Can you work these out from the model? Positions are in its coordinate system, mm. Face numbers are marked on the shaded views. Round coordinates to 2 decimals unless told otherwise and drop trailing zeros. Loops run counter-clockwise (first coordinate to the right, second up) from the corner with the lowest first, then second, coordinate; pieces in that order, holes last. Notation, with made-up numbers: (-18.5, -22) -> (14.5, -22) arc R13 ccw to (14.5, -8) -> close; hole circle Ø2 at (72, 18). An arc over 180 degrees is marked (long way). Use a Markdown table: item, result.
from build123d import *

# Parameters (mm, degrees)
F0_R     = 11.2
F0_R_2   = 13.2
F1_DEPTH = 7


with BuildPart() as f1:
    # F0 (on Top) → F1 (new body)
    with BuildSketch(Plane.XY):
        with BuildLine():
            ThreePointArc((10.232901, 19.541287), (12.436123, 23.454365), (13.2, 27.879616))
            ThreePointArc((13.2, 27.879616), (-4.186254, 40.398213), (-10.544739, 19.939308))
            ThreePointArc((-10.544739, 19.939308), (-0.252816, 14.682038), (10.232901, 19.541287))
        make_face()
        with Locations((0, 27.879616)):
            Circle(F0_R, mode=Mode.SUBTRACT)
        with BuildLine():
            ThreePointArc((-10.944456, -13.939808), (-14.094014, -5.382436), (-22.039701, -0.908691))
            ThreePointArc((-22.039701, -0.908691), (-35.700302, -20.319652), (-11.995578, -19.101666))
            ThreePointArc((-11.995578, -19.101666), (-11.209906, -16.573704), (-10.944456, -13.939808))
        make_face()
        with Locations((-24.144456, -13.939808)):
            Circle(F0_R, mode=Mode.SUBTRACT)
        with BuildLine():
            ThreePointArc((37.344456, -13.939808), (32.892752, -4.055107), (22.540317, -0.837643))
            ThreePointArc((22.540317, -0.837643), (12.841425, -7.122074), (11.8068, -18.632596))
            ThreePointArc((11.8068, -18.632596), (26.530137, -26.922432), (37.344456, -13.939808))
        make_face()
        with Locations((24.144456, -13.939808)):
            Circle(F0_R, mode=Mode.SUBTRACT)
        with BuildLine():
            ThreePointArc((10.232901, 19.541287), (-0.252816, 14.682038), (-10.544739, 19.939308))
            ThreePointArc((-10.544739, 19.939308), (-11.60274, 6.92967), (-22.039701, -0.908691))
            ThreePointArc((-22.039701, -0.908691), (-14.094014, -5.382436), (-10.944456, -13.939808))
            ThreePointArc((-10.944456, -13.939808), (-11.209906, -16.573704), (-11.995578, -19.101666))
            ThreePointArc((-11.995578, -19.101666), (-0.1999, -13.513102), (11.8068, -18.632596))
            ThreePointArc((11.8068, -18.632596), (12.841425, -7.122074), (22.540317, -0.837643))
            ThreePointArc((22.540317, -0.837643), (11.80264, 6.583433), (10.232901, 19.541287))
        make_face()
        Circle(F0_R_2, mode=Mode.SUBTRACT)
        Circle(F0_R_2)
        Circle(F0_R, mode=Mode.SUBTRACT)
    extrude(amount=F1_DEPTH)


solid = f1.part
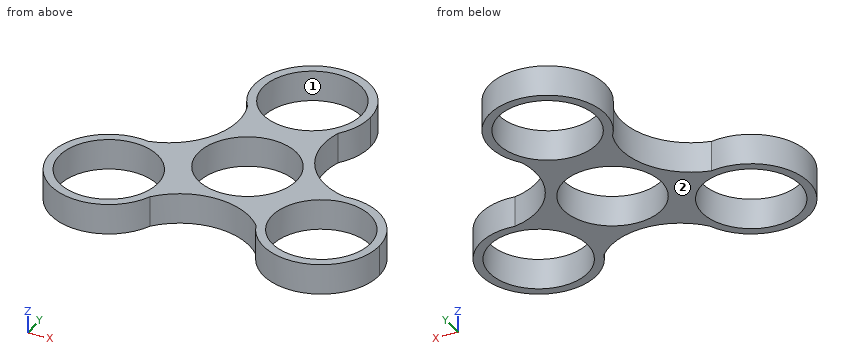
1. If we mould it in two halves opening along X, with no side actions, what happens to the marked faces 1 and 2? For each: +X half, -X half, draft (parallel to the pull), parting line (faces both ways), or undercut.
Answer sheet:
| item | result |
|---|---|
| face 1 | undercut |
| face 2 | draft |
2. I need wall thicknesses on line 1 (Y direction, x = 0, z = 6.5); line 2 (Y direction, x = -4.5, z = 2.25); line 3 (X direction, y = -6.5, z = 6.5). Which ranges of each line are inside material? Lowest first, please.
Answer sheet:
| item | result |
|---|---|
| line 1 | y = -13.51 to -11.2, 11.2 to 16.68, 39.08 to 41.08 |
| line 2 | y = -14.19 to -10.26, 10.26 to 17.62, 38.14 to 40.29 |
| line 3 | x = -35.05 to -32.52, -15.77 to -9.12, 9.12 to 15.77, 32.52 to 35.05 |
3. I want a section at D-D (y = -10). Please give me the cut outline in (x, z).
Answer sheet:
| item | result |
|---|---|
| outline | (-36.74, 0) -> (-34.63, 0) -> (-34.63, 7) -> (-36.74, 7) -> close; (-13.66, 0) -> (-5.04, 0) -> (-5.04, 7) -> (-13.66, 7) -> close; (5.04, 0) -> (13.66, 0) -> (13.66, 7) -> (5.04, 7) -> close; (34.63, 0) -> (36.74, 0) -> (36.74, 7) -> (34.63, 7) -> close |
4. I want a section at C-C (z = 5.5). Please give me the cut outline in (x, y), plus the area to 3 significant figures.
Answer sheet:
| item | result |
|---|---|
| outline | (-22.04, -0.91) arc R13.2 ccw (long way) to (-12, -19.1) arc R15.91 cw to (11.81, -18.63) arc R13.2 ccw (long way) to (22.54, -0.84) arc R15.91 cw to (10.23, 19.54) arc R13.2 ccw to (13.2, 27.88) arc R13.2 ccw (long way) to (-10.54, 19.94) arc R15.91 cw to start; hole circle Ø22.4 at (-24.14, -13.94); hole circle Ø22.4 at (0, 0); hole circle Ø22.4 at (0, 27.88); hole circle Ø22.4 at (24.14, -13.94) |
| area | 870 mm² |
5. Will these pins go through, and if not, where does the flat tip stop? pin 1 Ø2 at (y, z) = (-8.5, 4.5) entering from +X; pin 2 Ø1.5 at (x, z) = (21, 2) entering from +Y.
Answer sheet:
| item | result |
|---|---|
| pin 1 | stops at x = 36.58 |
| pin 2 | stops at y = -0.24 |
6. I want a section at B-B (x = 0). Please give me the cut outline in (y, z), plus the area to 3 significant figures.
Answer sheet:
| item | result |
|---|---|
| outline | (-13.51, 0) -> (-11.2, 0) -> (-11.2, 7) -> (-13.51, 7) -> close; (11.2, 0) -> (16.68, 0) -> (16.68, 7) -> (11.2, 7) -> close; (39.08, 0) -> (41.08, 0) -> (41.08, 7) -> (39.08, 7) -> close |
| area | 68.5 mm² |
7. I want a section at A-A (y = 23.5). Please give me the cut outline in (x, z), plus the area to 3 significant figures.
Answer sheet:
| item | result |
|---|---|
| outline | (-12.45, 0) -> (-10.31, 0) -> (-10.31, 7) -> (-12.45, 7) -> close; (10.31, 0) -> (12.45, 0) -> (12.45, 7) -> (10.31, 7) -> close |
| area | 30.0 mm² |
